```python
from build123d import *

# Parameters (mm, degrees)
F0_W     = 0.75
F0_H     = 1.75
F1_DEPTH = 8
F2_R     = 40
F3_R     = 20
F4_R     = 5
F5_R     = 2.5
F6_SIZE  = 2
F7_R     = 2.125
F8_DEPTH = 37.1109272381
F9_SIZE  = 0.75
F10_SIZE = 1


with BuildPart() as f1:
    # F0 (on Top) → F1 (new body)
    with BuildSketch(Plane.XY):
        Polygon((-10.75, -17), (-7.75, -17), (-7.75, -15.25), (-7.75, 0), (7.75, 0), (7.75, -15.25), (7.75, -17), (10.75, -17), (10.75, 0), (30.3688021535, 33.9807621135), (23.4405989232, 37.9807621135), (8.4405989232, 12), (-10.75, 12), align=None)
        with Locations((-7.375, -16.125)):
            Rectangle(F0_W, F0_H)
        with Locations((7.375, -16.125)):
            Rectangle(F0_W, F0_H)
    extrude(amount=F1_DEPTH)

    # F2
    f2_edges = [f1.edges().sort_by_distance(p)[0] for p in [
        (10.75, 0, 4),
    ]]
    fillet(f2_edges, radius=F2_R)

    # F3
    f3_edges = [f1.edges().sort_by_distance(p)[0] for p in [
        (8.440599, 12, 4),
    ]]
    fillet(f3_edges, radius=F3_R)

    # F4
    f4_edges = [f1.edges().sort_by_distance(p)[0] for p in [
        (-10.75, 12, 4),
    ]]
    fillet(f4_edges, radius=F4_R)

    # F5
    f5_edges = [f1.edges().sort_by_distance(p)[0] for p in [
        (10.75, -17, 4),
        (-10.75, -17, 4),
    ]]
    fillet(f5_edges, radius=F5_R)

    # F6
    f6_edges = [f1.edges().sort_by_distance(p)[0] for p in [
        (30.368802, 33.980762, 4),
        (23.440599, 37.980762, 4),
    ]]
    chamfer(f6_edges, length=F6_SIZE)

    # F7 (on face) → F8 (cut, through all)
    with BuildSketch(Plane(origin=(8.0625, -4.6548865453, 0), x_dir=(0.5, 0.8660254038, 0), z_dir=(0.8660254038, -0.5, 0))):
        with Locations((38.612604307, 4)):
            Circle(F7_R)
    extrude(amount=-F8_DEPTH, mode=Mode.SUBTRACT)

    # F9
    f9_edges = [f1.edges().sort_by_distance(p)[0] for p in [
        (18.32735, 29.124356, 8),
        (23.806624, 36.614737, 8),
        (6.893594, 14.679492, 8),
        (26.904701, 35.980762, 8),
        (-4.428203, 12, 8),
        (29.002777, 33.614737, 8),
        (-9.285534, 10.535534, 8),
        (22.738893, 20.765372, 8),
        (-10.75, -3.75, 8),
        (12.112967, -0.365206, 8),
        (-10.017767, -16.267767, 8),
        (10.75, -12.608984, 8),
        (-7.625, -17, 8),
        (10.017767, -16.267767, 8),
        (-7, -16.125, 8),
        (7.625, -17, 8),
        (-7.375, -15.25, 8),
        (7, -16.125, 8),
        (-7.75, -7.625, 8),
        (7.375, -15.25, 8),
        (0, 0, 8),
        (7.75, -7.625, 8),
        (18.32735, 29.124356, 0),
        (23.806624, 36.614737, 0),
        (6.893594, 14.679492, 0),
        (26.904701, 35.980762, 0),
        (-4.428203, 12, 0),
        (29.002777, 33.614737, 0),
        (-9.285534, 10.535534, 0),
        (22.738893, 20.765372, 0),
        (-10.75, -3.75, 0),
        (12.112967, -0.365206, 0),
        (-10.017767, -16.267767, 0),
        (10.75, -12.608984, 0),
        (-7.625, -17, 0),
        (10.017767, -16.267767, 0),
        (-7, -16.125, 0),
        (7.625, -17, 0),
        (-7.375, -15.25, 0),
        (7, -16.125, 0),
        (-7.75, -7.625, 0),
        (7.375, -15.25, 0),
        (0, 0, 0),
        (7.75, -7.625, 0),
    ]]
    chamfer(f9_edges, length=F9_SIZE)

    # F10
    f10_edges = [f1.edges().sort_by_distance(p)[0] for p in [
        (-7, -17, 4),
        (7, -17, 4),
    ]]
    chamfer(f10_edges, length=F10_SIZE)


solid = f1.part
```
Source: CAD feature listing. Evaluate the final solid. Frame: model axes, mm. Coordinates: 2 decimals unless noted, no trailing zeros. Write each loop counter-clockwise with the first axis right and the second up, starting at its lowest first coordinate (ties: lowest second). Pieces come first, ordered by that corner, then holes. Notation, with made-up numbers: (3, 35.5) -> (35, 35.5) arc R28 ccw to (35, 64.5) -> close; hole circle Ø8 at (87.5, 25.25). An arc over 180 degrees is marked (long way). Return JSON: item names as keys, results as strings. Group by question number.
1) Contact query for flat-ended pins moving along their axis: P1, Ø3, axis at y = 7.5, z = 4, coming from the -X side; P2, Ø0.6, axis at y = -15.5, z = 5.5, coming from the +X side; P3, Ø4, axis at x = 6, z = 2, coming from the +Y side; P4, Ø3, axis at x = -4, z = 4.5, coming from the +Y side. Output: stop coordinate, or through.
2) Section query B-B, the plane x = -5. Return loops of the section in (y, z), plus the area to 3 significant figures.
3) Section query A-A, the plane y = -12.5. Return loops of the section in (x, z), plus the area to 4 significant figures.
4) Ray query, line 1 along Y through (x, z) = (-4.5, 2); line 2 along X through (y, z) = (-6.5, 4.5); line 3 along Y through (x, z) = (24, 1). Return the intervals inside material, ascending.
5) Mould query, pull axis Y, two halves, no side actions, for faces 1 (the face through (24.93, 32.46, 3.19)), 2 (the face through (12.075, -0.507, 4.046)), 3 (the face through (-8.81, 10.12, 7.88)). Classes: +Y half, -Y half, draft (parallel to the pull), parting line (faces both ways), or undercut.
From the geometry:
{
 "1": {"P1": "x = -10.75", "P2": "x = 10.65", "P3": "y = 15.37", "P4": "y = 12.01"},
 "2": {"outline": "(0, 0.75) -> (0.75, 0) -> (11.25, 0) -> (12, 0.75) -> (12, 7.25) -> (11.25, 8) -> (0.75, 8) -> (0, 7.25) -> close", "area": "94.9 mm²"},
 "3": {"outline": "(-10.75, 0.75) -> (-10, 0) -> (-8.5, 0) -> (-7.75, 0.75) -> (-7.75, 7.25) -> (-8.5, 8) -> (-10, 8) -> (-10.75, 7.25) -> close; (7.75, 0.75) -> (8.5, 0) -> (10, 0) -> (10.75, 0.75) -> (10.75, 7.25) -> (10, 8) -> (8.5, 8) -> (7.75, 7.25) -> close", "area": "45.75 mm²"},
 "4": {"line 1": "0 to 12", "line 2": "-10.75 to -7.75, 7.75 to 10.97", "line 3": "22.95 to 36.67"},
 "5": {"face 1": "undercut", "face 2": "-Y half", "face 3": "+Y half"}
}
